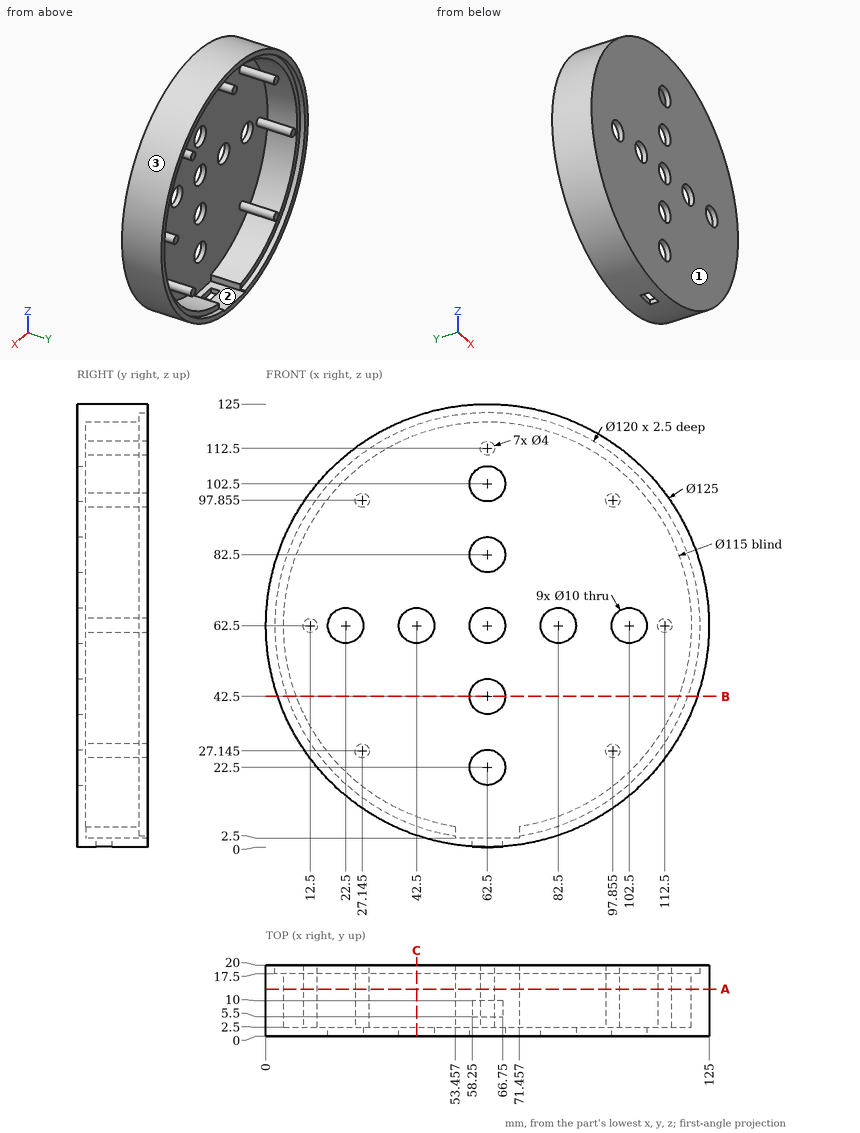
For this review, use the dimensioned drawing (mm, ordinates from the lowest corner) and the shaded views. Give positions to 0.01 mm unless a question says otherwise; leave off trailing zeros. Order: outer loops, then holes, each group sorted by start corner. A loop starts at its lowest first (then second) coordinate and runs counter-clockwise, first axis right, second up. Notation, with made-up numbers: (42, 8.5) -> (74, 8.5) arc R27 cw to (74, 41.5) -> close; hole circle Ø8 at (42, 34.25). An arc over 180 degrees is marked (long way). Write item = value, one per line. Start each with the question number.
(1) For pin 1 Ø12 at (x, z) = (69.5, 96) entering from +Y; pin 2 Ø3 at (x, y) = (35, 5.5) entering from -Z (1 decimal); pin 3 Ø9 at (x, z) = (62.5, 62.5) entering from +Y; pin 4 Ø1 at (y, z) = (10.5, 73) entering from -X (1 decimal), all flat-tipped, find the tip position at first contact; note any pin that passes through.
(2) Take a section at C-C (x = 42.5). Write out the cut boundary in (y, z).
(3) Draft analysis for pull direction Z (two halves, no side actions). For the marked faces 1, 2 and 3, state which applies: +Z half, -Z half, draft (parallel to the pull), parting line (faces both ways), or undercut.
(4) Take a section at B-B (z = 42.5). Write out the cut boundary in (x, y).
(5) Take a section at A-A (y = 13.25). State how many separate pieces and enclosed holes the cut face has, plus the area to 3 significant figures.
(6) For L1, parallel to Z at x = 62.5, y = 1.45; L2, parallel to Z at x = 62.5, y = 18.6; L3, parallel to X at y = 8, z = 25.5 (1 decimal), list the stretches that pass through material, from the lowest coordinate up. Write a range as from..to.
Returned:
q1.pin_1 = 2.5
q1.pin_2 = 5.7
q1.pin_3 = through
q1.pin_4 = 0.8
q2.outline = (0, 3.29) -> (20, 3.29) -> (20, 5.93) -> (17.5, 5.93) -> (17.5, 8.59) -> (2.5, 8.59) -> (2.5, 57.5) -> (0, 57.5) -> close; (0, 67.5) -> (2.5, 67.5) -> (2.5, 116.41) -> (17.5, 116.41) -> (17.5, 119.07) -> (20, 119.07) -> (20, 121.71) -> (0, 121.71) -> close
q3.face_1 = draft
q3.face_2 = undercut
q3.face_3 = parting line
q4.outline = (3.29, 0) -> (57.5, 0) -> (57.5, 2.5) -> (8.59, 2.5) -> (8.59, 17.5) -> (5.93, 17.5) -> (5.93, 20) -> (3.29, 20) -> close; (67.5, 0) -> (121.71, 0) -> (121.71, 20) -> (119.07, 20) -> (119.07, 17.5) -> (116.41, 17.5) -> (116.41, 2.5) -> (67.5, 2.5) -> close
q5.separate_pieces = 8
q5.enclosed_holes = 1
q5.area = 1,920 mm²
q6.L1 = 0..17.5, 27.5..37.5, 47.5..57.5, 67.5..77.5, 87.5..97.5, 107.5..125
q6.L2 = 0..2.5, 110.5..114.5, 122.5..125
q6.L3 = 12.1..18.5, 26..28.3, 96.7..99, 106.5..112.9
